Check sheet for the drawn part. Datum: minimum x, y, z corner. Units: mm. Give positions to 0.01 mm unless a question says otherwise; leave off trailing zeros. Loops run counter-clockwise (first coordinate to the right, second up) from the corner with the lowest first, then second, coordinate; pieces in that order, holes last. Notation, with made-up numbers: (-21.5, 9) -> (14.5, 9) arc R16 ccw to (14.5, 27) -> close; hole circle Ø11 at (-12, 60.5). An arc over 180 degrees is marked (long way). One line per question, with ' | ' between items.
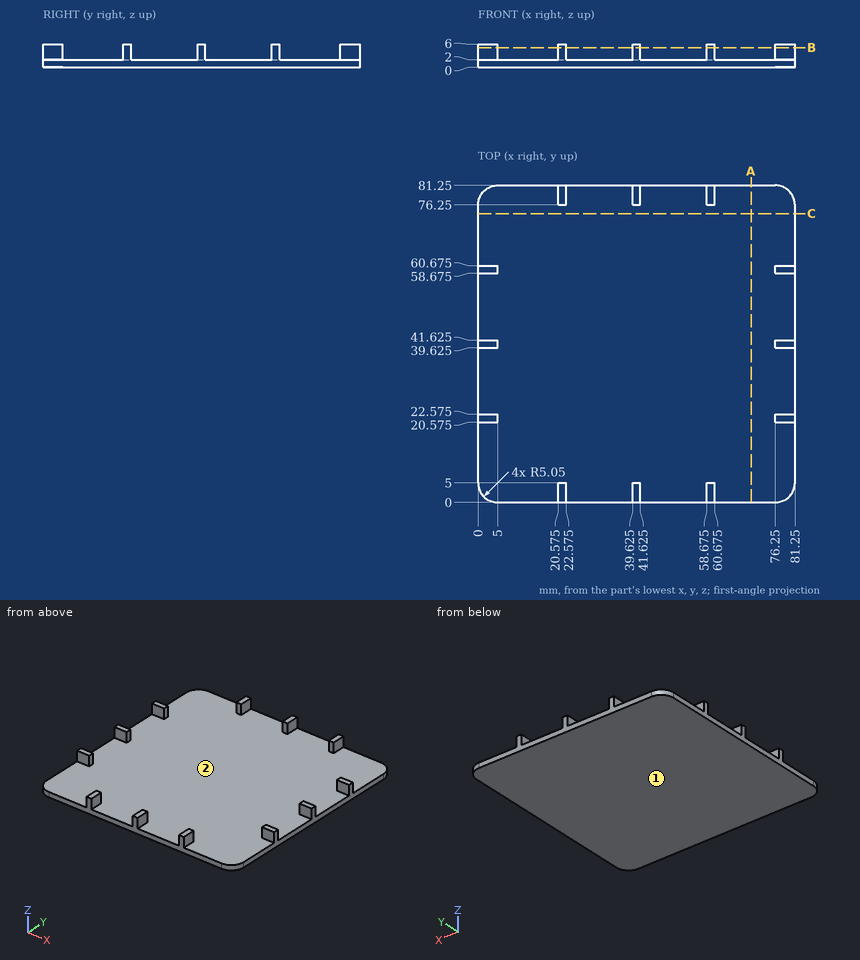
Item 1: Depth check by flat-ended pin: pin 1 Ø3 at (x, z) = (79, 4) entering from +Y (3 decimals); pin 2 Ø2 at (x, z) = (78.5, 4.5) entering from -Y (3 decimals); pin 3 Ø4 at (x, y) = (39.5, 28) entering from -Z; pin 4 Ø1.2 at (y, z) = (79, 4.5) entering from -X (3 decimals). Enter the tip coordinate at first touch or a pass-through.
Result:
pin 1: y = 60.675 | pin 2: y = 20.575 | pin 3: z = 0 | pin 4: x = 20.575
Item 2: Sectioned sample at A-A (x = 70). Record the cut outline in (y, z).
Result:
outline: (0, 0) -> (81.25, 0) -> (81.25, 2) -> (0, 2) -> close
Item 3: Scan lines: probe 1 along Y at (x, z) = (4.5, 3.1) (3 decimals); probe 2 along X at (y, z) = (60, 4.2). Record each from-to range of solid material in increasing order.
Result:
probe 1: 20.575 to 22.575, 39.625 to 41.625, 58.675 to 60.675 | probe 2: 0 to 5, 76.25 to 81.25
Item 4: Sectioned sample at B-B (z = 5.1). Give the number of separate pieces and of enclosed holes in the cut face, plus the area to 3 significant figures.
Result:
separate pieces: 12 | enclosed holes: 0 | area: 120 mm2
Item 5: Release check for a two-part mould opening along X. For the marked faces 1 and 2 record: pulls with the +X half, pulls with the -X half, needs draft (parallel to the pull), parting line crosses it, or undercut.
Result:
face 1: needs draft | face 2: undercut
